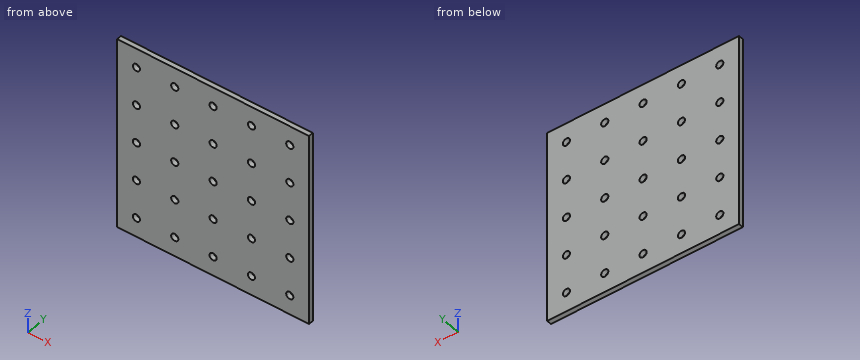
```python
from build123d import *

# Parameters (mm, degrees)
SKETCH1_W               = 127
SKETCH1_H               = 127
BOSS_EXTRUDE1_DEPTH     = 3.175
CUT_EXTRUDE3_DEPTH      = 3.175
CUT_EXTRUDE3_DEPTH_BACK = 90.858670283
SKETCH2_R               = 2.38125


with BuildPart() as part:
    # Sketch1 → Boss-Extrude1 (new body)
    with BuildSketch(Plane(origin=(0, 0, 0), x_dir=(1, 0, 0), z_dir=(0, 1, 0))):
        Rectangle(SKETCH1_W, SKETCH1_H)
    extrude(amount=BOSS_EXTRUDE1_DEPTH)

    # Sketch2 → Cut-Extrude3 (cut, two sides: drawn at the far end of the back side and taken through both)
    with BuildSketch(Plane(origin=(0, 0, 0), x_dir=(1, 0, 0), z_dir=(0, 1, 0)).offset(-CUT_EXTRUDE3_DEPTH_BACK)):
        with Locations(Location((-50.8, -50.8, 0), (0, 0, 270))):
            Circle(SKETCH2_R)
        with Locations(Location((-25.4, -50.8, 0), (0, 0, 270))):
            Circle(SKETCH2_R)
        with Locations(Location((0, -50.8, 0), (0, 0, 270))):
            Circle(SKETCH2_R)
        with Locations(Location((25.4, -50.8, 0), (0, 0, 270))):
            Circle(SKETCH2_R)
        with Locations(Location((50.8, -50.8, 0), (0, 0, 270))):
            Circle(SKETCH2_R)
        with Locations(Location((-25.4, -25.4, 0), (0, 0, 270))):
            Circle(SKETCH2_R)
        with Locations(Location((0, -25.4, 0), (0, 0, 270))):
            Circle(SKETCH2_R)
        with Locations(Location((25.4, -25.4, 0), (0, 0, 270))):
            Circle(SKETCH2_R)
        with Locations(Location((50.8, -25.4, 0), (0, 0, 270))):
            Circle(SKETCH2_R)
        with Locations(Location((-25.4, 0, 0), (0, 0, 270))):
            Circle(SKETCH2_R)
        with Locations(Location((0, 0, 0), (0, 0, 270))):
            Circle(SKETCH2_R)
        with Locations(Location((25.4, 0, 0), (0, 0, 270))):
            Circle(SKETCH2_R)
        with Locations(Location((50.8, 0, 0), (0, 0, 270))):
            Circle(SKETCH2_R)
        with Locations(Location((-25.4, 25.4, 0), (0, 0, 270))):
            Circle(SKETCH2_R)
        with Locations(Location((0, 25.4, 0), (0, 0, 270))):
            Circle(SKETCH2_R)
        with Locations(Location((25.4, 25.4, 0), (0, 0, 270))):
            Circle(SKETCH2_R)
        with Locations(Location((50.8, 25.4, 0), (0, 0, 270))):
            Circle(SKETCH2_R)
        with Locations(Location((-25.4, 50.8, 0), (0, 0, 270))):
            Circle(SKETCH2_R)
        with Locations(Location((0, 50.8, 0), (0, 0, 270))):
            Circle(SKETCH2_R)
        with Locations(Location((25.4, 50.8, 0), (0, 0, 270))):
            Circle(SKETCH2_R)
        with Locations(Location((50.8, 50.8, 0), (0, 0, 270))):
            Circle(SKETCH2_R)
        with Locations(Location((-50.8, -25.4, 0), (0, 0, 270))):
            Circle(SKETCH2_R)
        with Locations(Location((-50.8, 0, 0), (0, 0, 270))):
            Circle(SKETCH2_R)
        with Locations(Location((-50.8, 25.4, 0), (0, 0, 270))):
            Circle(SKETCH2_R)
        with Locations(Location((-50.8, 50.8, 0), (0, 0, 270))):
            Circle(SKETCH2_R)
    extrude(amount=CUT_EXTRUDE3_DEPTH + CUT_EXTRUDE3_DEPTH_BACK, mode=Mode.SUBTRACT)


solid = part.part
```
Input: part model. Units: mm. Frame: model coordinates. Coordinates: 2 decimals unless noted, no trailing zeros. Loops run counter-clockwise (first coordinate to the right, second up) from the corner with the lowest first, then second, coordinate; pieces in that order, holes last. Notation, with made-up numbers: M -1,88.5 L 34,88.5 A32 ccw 34,123.5 Z; hole C 12,68 d3. An arc over 180 degrees is marked long. Use a Markdown table: item, result. Add a question column.
1) Section B-B, the plane y = 2.1. Give the number of separate pieces and of enclosed holes in the cut face, plus the area to 3 significant figures.
2) Pin query (flat end, axial travel): P1, Ø3, axis at x = 50.8, z = 50.8, coming from the +Y side. Return the tip coordinate at first contact, or that it passes through.
3) Section A-A, the plane x = -50.8. Return the cut outline in (y, z) (3 decimals), plus the area to 3 significant figures.
4) Section C-C, the plane z = -25.4. Return the cut outline in (x, y) (3 decimals), plus the area to 3 significant figures.
5) Line query: L1, parallel to X at y = 1.6, z = 50.8; L2, parallel to Z at x = 24.5, y = 0.9. Output: solid intervals per line, ascending. Write a range as from..to.
Answer below:
| question | item | result |
|---|---|---|
| 1 | separate pieces | 1 |
| 1 | enclosed holes | 25 |
| 1 | area | 15,700 mm2 |
| 2 | P1 | through |
| 3 | outline | M 0,-63.5 L 3.175,-63.5 L 3.175,-53.181 L 0,-53.181 Z; M 0,-48.419 L 3.175,-48.419 L 3.175,-27.781 L 0,-27.781 Z; M 0,-23.019 L 3.175,-23.019 L 3.175,-2.381 L 0,-2.381 Z; M 0,2.381 L 3.175,2.381 L 3.175,23.019 L 0,23.019 Z; M 0,27.781 L 3.175,27.781 L 3.175,48.419 L 0,48.419 Z; M 0,53.181 L 3.175,53.181 L 3.175,63.5 L 0,63.5 Z |
| 3 | area | 328 mm2 |
| 4 | outline | M -63.5,0 L -53.181,0 L -53.181,3.175 L -63.5,3.175 Z; M -48.419,0 L -27.781,0 L -27.781,3.175 L -48.419,3.175 Z; M -23.019,0 L -2.381,0 L -2.381,3.175 L -23.019,3.175 Z; M 2.381,0 L 23.019,0 L 23.019,3.175 L 2.381,3.175 Z; M 27.781,0 L 48.419,0 L 48.419,3.175 L 27.781,3.175 Z; M 53.181,0 L 63.5,0 L 63.5,3.175 L 53.181,3.175 Z |
| 4 | area | 328 mm2 |
| 5 | L1 | -63.5..-53.18, -48.42..-27.78, -23.02..-2.38, 2.38..23.02, 27.78..48.42, 53.18..63.5 |
| 5 | L2 | -63.5..-53, -48.6..-27.6, -23.2..-2.2, 2.2..23.2, 27.6..48.6, 53..63.5 |
